```python
from build123d import *

# Parameters (mm, degrees)
F0_W     = 1500
F0_H     = 600
F1_DEPTH = 1200
F3_DEPTH = 1600
F4_W     = 350
F4_H     = 700
F5_DEPTH = 1500
F6_W     = 330
F6_H     = 420
F7_DEPTH = 2000
F8_W     = 653.322876
F8_H     = 64.883091
F9_DEPTH = 1500


with BuildPart() as f1:
    # F0 (on Top) → F1 (new body)
    with BuildSketch(Plane.XY):
        Rectangle(F0_W, F0_H)
    extrude(amount=F1_DEPTH)

    # F2 (on face) → F3 (cut)
    with BuildSketch(Plane.YZ.offset(750)):
        with BuildLine():
            ThreePointArc((-300, 804.887652), (-59.205292, 1092.350344), (300, 1200))
            Line((300, 1200), (-300, 1200))
            Line((-300, 1200), (-300, 804.887652))
        make_face()
    extrude(amount=-F3_DEPTH, mode=Mode.SUBTRACT)

    # F4 (on face) → F5 (cut)
    with BuildSketch(Plane.XZ.offset(300)):
        with Locations((-575, 350)):
            Rectangle(F4_W, F4_H)
        with Locations((575, 350)):
            Rectangle(F4_W, F4_H)
    extrude(amount=-F5_DEPTH, mode=Mode.SUBTRACT)

    # F6 (on face) → F7 (cut)
    with BuildSketch(Plane.XZ.offset(300)):
        with Locations((-585, 1014.887652)):
            Rectangle(F6_W, F6_H)
        with Locations((585, 1014.887652)):
            Rectangle(F6_W, F6_H)
    extrude(amount=-F7_DEPTH, mode=Mode.SUBTRACT)

    # F8 (on face) → F9 (cut)
    with BuildSketch(Plane.XZ.offset(300)):
        with Locations((12.039125, 32.441545)):
            Rectangle(F8_W, F8_H)
    extrude(amount=-F9_DEPTH, mode=Mode.SUBTRACT)


solid = f1.part
```
Part model, mm, in its own coordinate system. A direction names the side the tool comes from. Round coordinates to 2 decimals unless told otherwise and drop trailing zeros. Loops run counter-clockwise (first coordinate to the right, second up) from the corner with the lowest first, then second, coordinate; pieces in that order, holes last. Notation, with made-up numbers: (62, 62.25) -> (102, 62.25) arc R24 ccw to (102, 76.25) -> close; hole circle Ø5 at (34, 84). An arc over 180 degrees is marked (long way). Use CSV: the item, a comma, the result in double quotes. Start each with the question number.
1) Cut at B-B, the plane z = 593. Write the cut outline in (x, y).
2) Drop flat-ended pins along their axis: P1, Ø4, axis at y = 172.5, z = 1007, coming from the -X side; P2, Ø1.5, axis at x = -143, y = -134, coming from the +Z side; P3, Ø4, axis at x = 291, y = -230, coming from the +Z side. Give the stop position or say it passes through.
3) Cut at C-C, the plane x = -119. Write the cut outline in (y, z), plus the area to 3 significant figures.
4) Cut at D-D, the plane y = -22. Write the cut outline in (x, z), plus the area to 3 significant figures.
5) Cut at A-A, the plane y = -146. Write the cut outline in (x, z).
6) Wall check: L1, parallel to X at y = -187, z = 561; L2, parallel to Z at x = 422.5, y = -16.5; L3, parallel to X at y = 38, z = 987. Give the ranges that are in metal, low to high. Write a range as [from, to].
7) Which spindle directions (+Z, -Z, +X, -X, +Y, -Y) get a long thin tool onto all of the face, cutting with end or side? Do faces 1 (the flat face through (-314.622, -4, 32)), 2 (the flat face through (420, 62, 956)), 3 (the flat face through (-420, 62, 956)), 4 (the flat face through (-577, -4, 700)). Say none if no direction does.
Determined:
1,outline,"(-400, -300) -> (400, -300) -> (400, 300) -> (-400, 300) -> close"
2,P1,"stops at x = -420"
2,P2,"stops at z = 1035.61"
2,P3,"stops at z = 931.31"
3,outline,"(-300, 64.88) -> (300, 64.88) -> (300, 1200) arc R653.12 ccw to (-300, 804.89) -> close"
3,area,"615,000 mm2"
4,outline,"(-750, 700) -> (-400, 700) -> (-400, 0) -> (-314.62, 0) -> (-314.62, 64.88) -> (338.7, 64.88) -> (338.7, 0) -> (400, 0) -> (400, 700) -> (750, 700) -> (750, 804.89) -> (420, 804.89) -> (420, 1115.11) -> (-420, 1115.11) -> (-420, 804.89) -> (-750, 804.89) -> close"
4,area,"936,000 mm2"
5,outline,"(-750, 700) -> (-400, 700) -> (-400, 0) -> (-314.62, 0) -> (-314.62, 64.88) -> (338.7, 64.88) -> (338.7, 0) -> (400, 0) -> (400, 700) -> (750, 700) -> (750, 804.89) -> (420, 804.89) -> (420, 1024.01) -> (-420, 1024.01) -> (-420, 804.89) -> (-750, 804.89) -> close"
6,L1,"x = [-400, 400]"
6,L2,"z = [700, 804.89]"
6,L3,"x = [-420, 420]"
7,face 1,"-Z, +Y, -Y"
7,face 2,"+Z, +X, +Y, -Y"
7,face 3,"+Z, -X, +Y, -Y"
7,face 4,"-Z, -X, +Y, -Y"
